The figure shows three views and two pictorial views of one solid part (mm, origin at its lowest corner). Answer the questions. Round coordinates to 2 decimals unless told otherwise and drop trailing zeros. Order: outer loops, then holes, each group sorted by start corner. A loop starts at its lowest first (then second) coordinate and runs counter-clockwise, first axis right, second up. Notation, with made-up numbers: (57, 61) -> (113, 61) arc R24 ccw to (113, 77) -> close; hole circle Ø2 at (35.25, -18.5). An arc over 180 degrees is marked (long way). Answer as a JSON object with one key per item and string values. Group by question number.
Item 1: Given P1, Ø3, axis at x = 5, z = 2, coming from the -Y side; P2, Ø1.5, axis at y = 0.5, z = 6, coming from the +X side; P3, Ø5, axis at x = 7.94, z = 7.94, coming from the -Y side; P4, Ø6, axis at x = 12.5, z = 1.5, coming from the +Y side, each flat-ended and moving along its own axis, determine where each tip first touches the part or whether it passes through.
Item 2: Section D-D, the plane z = 11.5 is taken. Write down the section's boundary in (x, y) (1 decimal).
Item 3: Section A-A, the plane z = 5 is taken. Write down the section's boundary in (x, y).
Item 4: The mould has two halves that part along X. Classify the marked faces 1, 2 and 3: pulls with the +X half, pulls with the -X half, needs draft (parallel to the pull), parting line crosses it, or undercut.
Item 5: Section B-B, the plane x = 9.5 is taken. Write down the section's boundary in (y, z) (1 decimal).
Item 6: Consider probe 1 along Z at (x, y) = (8, 5.3) (1 decimal); probe 2 along Y at (x, z) = (9, 2). Determine where each line is inside the solid, lowest interval first. Write a range as from..to.
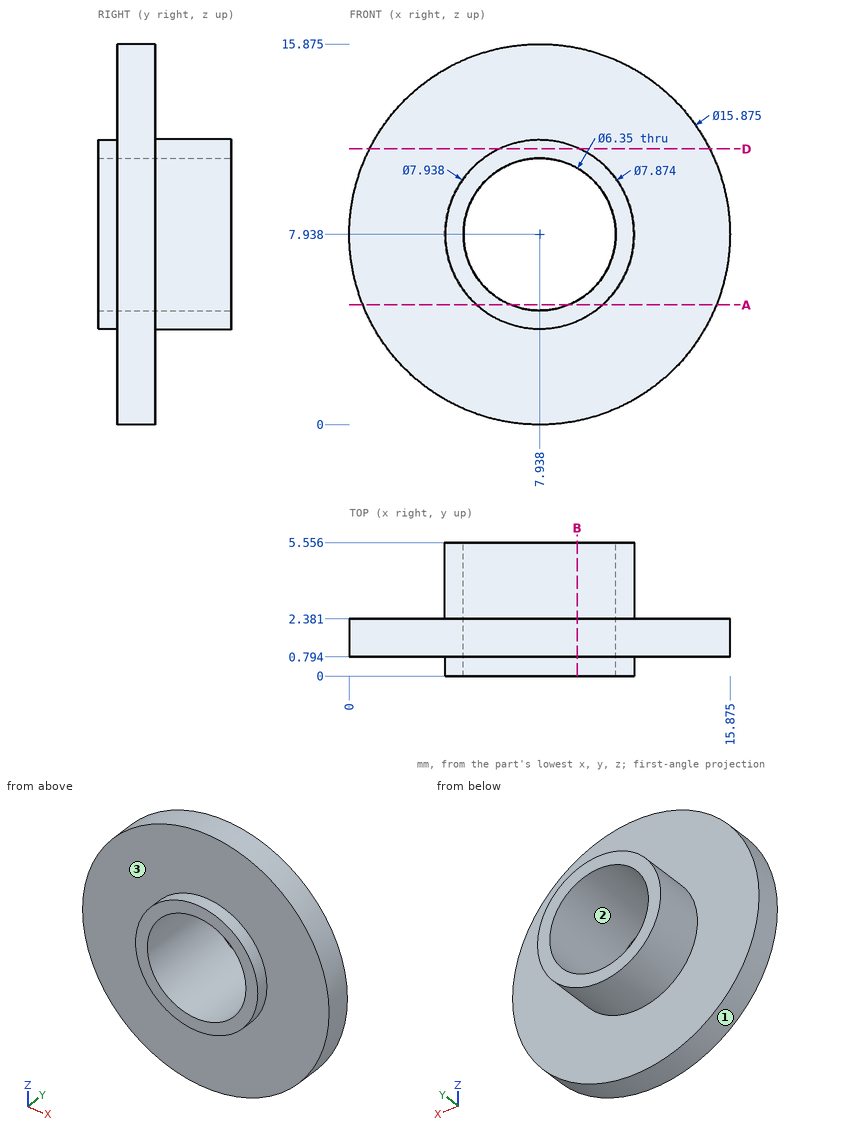
Values found:
{
 "1": {"P1": "y = 0.79", "P2": "x = 15.78", "P3": "through", "P4": "y = 2.38"},
 "2": {"outline": "(0.8, 0.8) -> (6.3, 0.8) -> (6.3, 0) -> (9.6, 0) -> (9.6, 0.8) -> (15, 0.8) -> (15, 2.4) -> (9.7, 2.4) -> (9.7, 5.6) -> (6.2, 5.6) -> (6.2, 2.4) -> (0.8, 2.4) -> close"},
 "3": {"outline": "(0.56, 0.79) -> (5.32, 0.79) -> (5.32, 0) -> (6.73, 0) -> (6.73, 5.56) -> (5.27, 5.56) -> (5.27, 2.38) -> (0.56, 2.38) -> close; (9.14, 0) -> (10.56, 0) -> (10.56, 0.79) -> (15.31, 0.79) -> (15.31, 2.38) -> (10.61, 2.38) -> (10.61, 5.56) -> (9.14, 5.56) -> close"},
 "4": {"face 1": "parting line crosses it", "face 2": "undercut", "face 3": "needs draft"},
 "5": {"outline": "(0, 4.3) -> (0.8, 4.3) -> (0.8, 0.2) -> (2.4, 0.2) -> (2.4, 4.3) -> (5.6, 4.3) -> (5.6, 5.2) -> (0, 5.2) -> close; (0, 10.7) -> (5.6, 10.7) -> (5.6, 11.6) -> (2.4, 11.6) -> (2.4, 15.7) -> (0.8, 15.7) -> (0.8, 11.6) -> (0, 11.6) -> close"},
 "6": {"probe 1": "4..4.8, 11.1..11.9", "probe 2": "0.79..2.38"}
}
